The model under review builds one solid part; all positions refer to its coordinate system, in mm. Give positions to 0.01 mm unless a question says otherwise; leave off trailing zeros. Write each loop counter-clockwise with the first axis right and the second up, starting at its lowest first coordinate (ties: lowest second). Pieces come first, ordered by that corner, then holes. Notation, with made-up numbers: M -35,-39 L -7,-39 A13 cw -7,-14 Z; hole C 73,46 d10. An arc over 180 degrees is marked long. Write item = value, one per line. Start each with the question number.
Autodesk Inventor part; units mm, degrees
ref_plane "YZ Plane" through (0, 0, 0) normal (1, 0, 0) x (0, 1, 0)
ref_plane "XZ Plane" through (0, 0, 0) normal (0, 1, 0) x (-1, 0, 0)
ref_plane "XY Plane" through (0, 0, 0) normal (0, 0, 1) x (1, 0, 0)
sketch "Sketch1" plane through (0, 0, 0) normal (0, 0, 1) x (1, 0, 0)
  line L0 (0, 0) -> (-15, 0)
  line L1 (-15, 0) -> (-15, 50)
  line L2 (-15, 50) -> (-5, 50)
  line L3 (-5, 50) -> (0, 0)
  dimension "d0" = 10
  dimension "d1" = 50
  dimension "d16" = 15
extrude "Extrusion1" add sketch "Sketch1" along normal blind 5
sketch "Sketch2" plane through (0, 0, 5) normal (0, 0, 1) x (1, 0, 0)
  line L0 (-15, 50) -> (-15, 0)
  line L1 (-5, 50) -> (-15, 50)
  line L2 (-15, 0) -> (0, 0)
  point P0 (-10, 42.5)
  point P1 (-10, 7.5)
  dimension "d6" = 7.5
  dimension "d7" = 7.5
  dimension "d8" = 35
  dimension "d17" = 5
hole "Hole1" at (-10, 42.5, 5) at (-10, 7.5, 5) direction (0, 0, -1) diameter 4.5 end through all countersink diameter 9.4 countersink angle 90
properties part number "Pancake_Side Piece Short 3" material "Wood (Birch)"
Item 1: We need section A-A, the plane y = 42.5. Write out the cut boundary in (x, z).
Item 2: We need section B-B, the plane x = -10. Write out the cut boundary in (y, z).
Item 3: We need section D-D, the plane y = 7.5. Write out the cut boundary in (x, z).
Item 4: Clearance check with a flat-ended pin moving along its axis: P1, Ø7, axis at x = -10, y = 42.5, coming from the -Z side. State where the tip first meets the part, or that it passes through.
Item 5: The part is to be moulded in two halves that separate along Y. For faces 1 (the flat face through (-10, 50, 2)), 2 (the flat face through (-9, 25, 0)), 3 (the cylindrical face through (-11.52, 9.16, 1.26)), say which applies: released by +Y, released by -Y, zero draft, split by the parting line, or undercut.
Item 6: To check wall thickness, follow probe 1 along Y at (x, z) = (-10, 0.6); probe 2 along Y at (x, z) = (-8.5, 1.85); probe 3 along X at (y, z) = (7.5, 1.45). State the ranges of each line that lie inside material, in increasing order. Write a range as [from, to].
Item 7: We need section C-C, the plane z = 4. Write out the cut boundary in (x, y).
Worked out:
q1.outline = M -15,0 L -12.25,0 L -12.25,2.55 L -14.7,5 L -15,5 Z; M -7.75,0 L -4.25,0 L -4.25,5 L -5.3,5 L -7.75,2.55 Z
q2.outline = M 0,0 L 5.25,0 L 5.25,2.55 L 2.8,5 L 0,5 Z; M 9.75,0 L 40.25,0 L 40.25,2.55 L 37.8,5 L 12.2,5 L 9.75,2.55 Z; M 44.75,0 L 50,0 L 50,5 L 47.2,5 L 44.75,2.55 Z
q3.outline = M -15,0 L -12.25,0 L -12.25,2.55 L -14.7,5 L -15,5 Z; M -7.75,0 L -0.75,0 L -0.75,5 L -5.3,5 L -7.75,2.55 Z
q4.P1 = 0
q5.face_1 = released by +Y
q5.face_2 = zero draft
q5.face_3 = undercut
q6.probe_1 = [0, 5.25], [9.75, 40.25], [44.75, 50]
q6.probe_2 = [0, 5.82], [9.18, 40.82], [44.18, 50]
q6.probe_3 = [-15, -12.25], [-7.75, -0.75]
q7.outline = M -15,0 L 0,0 L -5,50 L -15,50 Z; hole C -10,7.5 d7.4; hole C -10,42.5 d7.4
